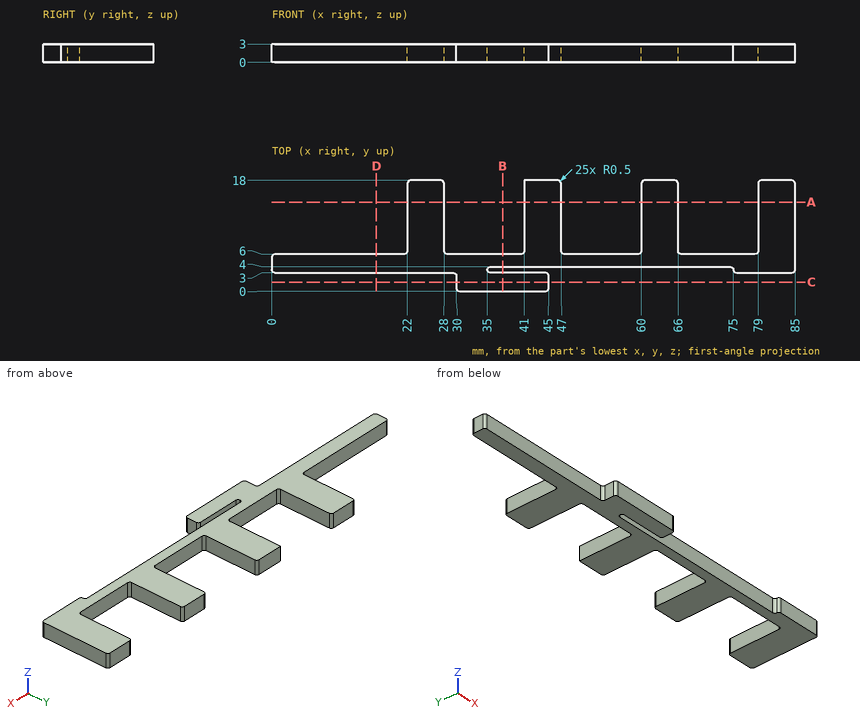
Check sheet for the drawn part. Datum: minimum x, y, z corner. Units: mm. Round coordinates to 2 decimals unless told otherwise and drop trailing zeros. Loops run counter-clockwise (first coordinate to the right, second up) from the corner with the lowest first, then second, coordinate; pieces in that order, holes last.
Item 1: Cross-section at B-B on x = 37.5. Record the boundary of the cut face in (y, z), then the cut area to 3 significant figures.
Item 2: Cross-section at C-C on y = 1.5. Record the boundary of the cut face in (x, z), then the cut area to 3 significant figures.
Item 3: Gauge pin test, flat ends, axial feed: pin 1 (0.9 mm diameter, centred on x = 80, z = 2, fed in from -Y); pin 2 (0.9 mm diameter, centred on x = 38, z = 2, fed in from +Y); pin 3 (0.9 mm diameter, centred on y = 10, z = 2, fed in from -X); pin 4 (1 mm diameter, centred on x = 13, y = 2, fed in from -Z). Record the tip position at first contact, or that the pin passes through.
Item 4: Thickness scan on line 1 (X direction, y = 12.5, z = 2.8); line 2 (Y direction, x = 38, z = 0.7); line 3 (Y direction, x = 13.5, z = 1.8). Record the ranges inside material, lowest first.
Item 5: Cross-section at D-D on x = 17. Record the boundary of the cut face in (y, z).
Item 6: Cross-section at A-A on y = 14.5. Record the boundary of the cut face in (x, z), then the cut area to 3 significant figures.
Answer sheet:
1. outline: (0, 0) - (3, 0) - (3, 3) - (0, 3) - close; (4, 0) - (6, 0) - (6, 3) - (4, 3) - close
1. area: 15.0 mm2
2. outline: (30, 0) - (45, 0) - (45, 3) - (30, 3) - close
2. area: 45.0 mm2
3. pin 1: stops at y = 3
3. pin 2: stops at y = 6
3. pin 3: stops at x = 22
3. pin 4: passes through
4. line 1: x = 22 to 28, 41 to 47, 60 to 66, 79 to 85
4. line 2: y = 0 to 3, 4 to 6
4. line 3: y = 3 to 6
5. outline: (3, 0) - (6, 0) - (6, 3) - (3, 3) - close
6. outline: (22, 0) - (28, 0) - (28, 3) - (22, 3) - close; (41, 0) - (47, 0) - (47, 3) - (41, 3) - close; (60, 0) - (66, 0) - (66, 3) - (60, 3) - close; (79, 0) - (85, 0) - (85, 3) - (79, 3) - close
6. area: 72.0 mm2
